```python
from build123d import *

# Parameters (mm, degrees)
F0_R     = 101.6
F1_DEPTH = 76.2
F2_R     = 50.8
F3_DEPTH = 127
F5_DEPTH = 127


with BuildPart() as f1:
    # F0 (on Top) → F1 (new body)
    with BuildSketch(Plane.XY):
        Circle(F0_R)
    extrude(amount=F1_DEPTH)

    # F2 (on face) → F3 (join)
    with BuildSketch(Plane.XY.offset(76.2)):
        Circle(F2_R)
    extrude(amount=F3_DEPTH)

    # F4 (on face) → F5 (join)
    with BuildSketch(Plane.XY.offset(203.2)):
        with BuildLine():
            Line((43.994091, 25.4), (-43.994091, 25.4))
            ThreePointArc((-43.994091, 25.4), (-50.8, 0), (-43.994091, -25.4))
            Line((-43.994091, -25.4), (43.994091, -25.4))
            ThreePointArc((43.994091, -25.4), (49.069032, -13.148007), (50.8, 0))
            ThreePointArc((50.8, 0), (49.069032, 13.148007), (43.994091, 25.4))
        make_face()
    extrude(amount=F5_DEPTH)


solid = f1.part
```
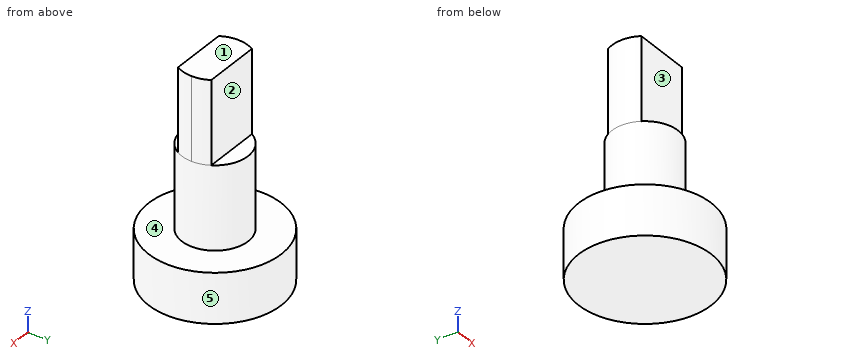
The model under review builds one solid part; all positions refer to its coordinate system, in mm. Face numbers are marked on the shaded views. A direction names the side the tool comes from. Round coordinates to 2 decimals unless told otherwise and drop trailing zeros. Order: outer loops, then holes, each group sorted by start corner. A loop starts at its lowest first (then second) coordinate and runs counter-clockwise, first axis right, second up. Notation, with made-up numbers: M 82,-25.5 L 118,-25.5 A14 ccw 118,-5.5 Z; hole C 79,20 d10. An arc over 180 degrees is marked long. Use a Markdown table: item, result.
1) Tool access review of the marked faces 1, 2, 3, 4 and 5: name each direction out of +Z, -Z, +X, -X, +Y, -Y from which nothing blocks a thin tool from reaching the whole face with its end or side.
Report:
| item | result |
|---|---|
| face 1 | +Z, +X, -X, +Y, -Y |
| face 2 | +Z, +X, -X, +Y |
| face 3 | +Z, +X, -X, -Y |
| face 4 | +Z |
| face 5 | +Z, -Z |
2) Consider section D-D (y = -37). Write out the cut boundary in (x, z), then the cut area to 3 significant figures.
Report:
| item | result |
|---|---|
| outline | M -94.62,0 L 94.62,0 L 94.62,76.2 L 34.81,76.2 L 34.81,203.2 L -34.81,203.2 L -34.81,76.2 L -94.62,76.2 Z |
| area | 23,300 mm^2 |
3) Insertion check: pin 1 (6 mm diameter, centred on x = -26, z = 57.5, fed in from -Y); pin 2 (2 mm diameter, centred on x = 30.5, y = 41, fed in from +Z); pin 3 (8 mm diameter, centred on x = -31, z = 136.5, fed in from -Y); pin 4 (5 mm diameter, centred on y = 28.5, z = 296, fed in from +X). Each pin has a flat end and moves straight along its axis. Give the tip position at first contact, or say it passes through.
Report:
| item | result |
|---|---|
| pin 1 | y = -98.96 |
| pin 2 | z = 203.2 |
| pin 3 | y = -43.03 |
| pin 4 | through |
4) Consider section C-C (z = 233.5). Write out the cut boundary in (x, y).
Report:
| item | result |
|---|---|
| outline | M -43.99,-25.4 L 43.99,-25.4 A50.8 ccw 50.8,0 A50.8 ccw 43.99,25.4 L -43.99,25.4 A50.8 ccw Z |
5) Consider section A-A (x = 0). Write out the cut boundary in (y, z).
Report:
| item | result |
|---|---|
| outline | M -101.6,0 L 101.6,0 L 101.6,76.2 L 50.8,76.2 L 50.8,203.2 L 25.4,203.2 L 25.4,330.2 L -25.4,330.2 L -25.4,203.2 L -50.8,203.2 L -50.8,76.2 L -101.6,76.2 Z |
6) Wall thickness on line 1 along Y through (x, z) = (-10, 254); line 2 along Z through (x, y) = (-84, -18); line 3 along Z through (x, y) = (33, 38.5): over which ranges is each line inside the solid? List them lowest first. Write a range as [from, to].
Report:
| item | result |
|---|---|
| line 1 | [-25.4, 25.4] |
| line 2 | [0, 76.2] |
| line 3 | [0, 203.2] |
7) Consider section B-B (y = 29). Write out the cut boundary in (x, z).
Report:
| item | result |
|---|---|
| outline | M -97.37,0 L 97.37,0 L 97.37,76.2 L 41.71,76.2 L 41.71,203.2 L -41.71,203.2 L -41.71,76.2 L -97.37,76.2 Z |
